Can you work these out from the model? Positions are in its coordinate system, mm. Round coordinates to 2 decimals unless told otherwise and drop trailing zeros. Write each loop counter-clockwise with the first axis right and the second up, starting at its lowest first coordinate (ties: lowest second). Pieces come first, ordered by that corner, then holes. Notation, with made-up numbers: M -15,29.5 L 0,29.5 A25 ccw 0,68.5 Z; hole C 34,-32.75 d10. An arc over 180 degrees is marked long. Answer in a Markdown table with one row per item. Add a question column.
(1) Suppose I cut it at B-B, the plane z = -16.5. Write out the boundary of the cut face in (x, y).
(2) Suppose I cut it at A-A, the plane x = -39. Write out the boundary of the cut face in (y, z), then the cut area to 3 significant figures.
(3) I'm going to push flat-ended pins straight in: pin 1 (1.5 mm diameter, centred on x = 27.5, y = 1, fed in from +Z); pin 2 (1.3 mm diameter, centred on x = -55.5, y = 1, fed in from -Z); pin 3 (1.3 mm diameter, centred on y = 2, z = -1, fed in from -X). Where does each tip first touch, or does it pass through?
(4) If I drill on probe 1 along X at (y, z) = (1.2, -22); probe 2 along X at (y, z) = (1.45, 20.5); probe 3 along Z at (x, y) = (-6, 0.25), over which ranges is the centre line in solid material (lowest first)?
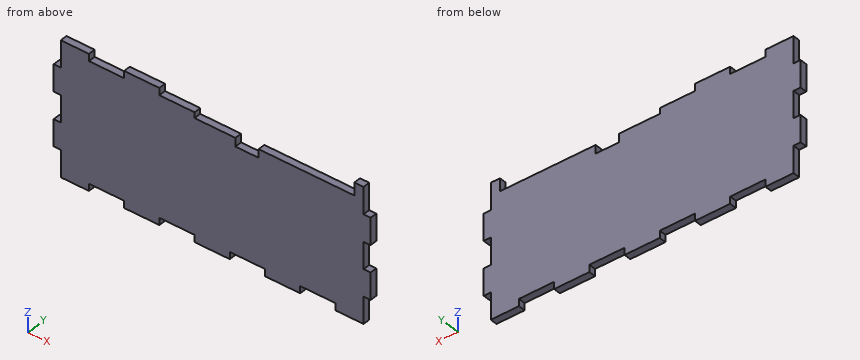
from build123d import *

# Parameters (mm, degrees)
SKETCH1_W           = 114.3
SKETCH1_H           = 48.006
BOSS_EXTRUDE1_DEPTH = 2.54
CUT_EXTRUDE2_REACH  = 64.038
SKETCH2_W           = 2.54
SKETCH2_H           = 9.6012
SKETCH2_W_2         = 12.7
SKETCH2_H_2         = 2.54
CUT_EXTRUDE3_DEPTH  = 2.54


with BuildPart() as part:
    # Sketch1 → Boss-Extrude1 (new body)
    with BuildSketch(Plane(origin=(0, 0, 0), x_dir=(1, 0, 0), z_dir=(0, 1, 0))):
        Rectangle(SKETCH1_W, SKETCH1_H)
    extrude(amount=BOSS_EXTRUDE1_DEPTH)

    # Sketch2 → Cut-Extrude2 (cut, up to next)
    with BuildSketch(Plane(origin=(0, 2.54, 0), x_dir=(1, 0, 0), z_dir=(0, 1, 0)), mode=Mode.PRIVATE) as cut_extrude2_sk1:
        with Locations((-55.88, 19.2024)):
            Rectangle(SKETCH2_W, SKETCH2_H)
    cut_extrude2_tool1 = extrude(cut_extrude2_sk1.sketch, amount=-CUT_EXTRUDE2_REACH, mode=Mode.PRIVATE) & part.part
    # Sketch2 → Cut-Extrude2 (cut, up to next)
    with BuildSketch(Plane(origin=(0, 2.54, 0), x_dir=(1, 0, 0), z_dir=(0, 1, 0)), mode=Mode.PRIVATE) as cut_extrude2_sk2:
        with Locations((-38.1, 22.733)):
            Rectangle(SKETCH2_W_2, SKETCH2_H_2)
    cut_extrude2_tool2 = extrude(cut_extrude2_sk2.sketch, amount=-CUT_EXTRUDE2_REACH, mode=Mode.PRIVATE) & part.part
    # Sketch2 → Cut-Extrude2 (cut, up to next)
    with BuildSketch(Plane(origin=(0, 2.54, 0), x_dir=(1, 0, 0), z_dir=(0, 1, 0)), mode=Mode.PRIVATE) as cut_extrude2_sk3:
        with Locations((-12.7, 22.733)):
            Rectangle(SKETCH2_W_2, SKETCH2_H_2)
    cut_extrude2_tool3 = extrude(cut_extrude2_sk3.sketch, amount=-CUT_EXTRUDE2_REACH, mode=Mode.PRIVATE) & part.part
    # Sketch2 → Cut-Extrude2 (cut, up to next)
    with BuildSketch(Plane(origin=(0, 2.54, 0), x_dir=(1, 0, 0), z_dir=(0, 1, 0)), mode=Mode.PRIVATE) as cut_extrude2_sk4:
        with Locations((12.7, 22.733)):
            Rectangle(SKETCH2_W_2, SKETCH2_H_2)
    cut_extrude2_tool4 = extrude(cut_extrude2_sk4.sketch, amount=-CUT_EXTRUDE2_REACH, mode=Mode.PRIVATE) & part.part
    # Sketch2 → Cut-Extrude2 (cut, up to next)
    with BuildSketch(Plane(origin=(0, 2.54, 0), x_dir=(1, 0, 0), z_dir=(0, 1, 0)), mode=Mode.PRIVATE) as cut_extrude2_sk5:
        with Locations((38.1, 22.733)):
            Rectangle(SKETCH2_W_2, SKETCH2_H_2)
    cut_extrude2_tool5 = extrude(cut_extrude2_sk5.sketch, amount=-CUT_EXTRUDE2_REACH, mode=Mode.PRIVATE) & part.part
    # Sketch2 → Cut-Extrude2 (cut, up to next)
    with BuildSketch(Plane(origin=(0, 2.54, 0), x_dir=(1, 0, 0), z_dir=(0, 1, 0)), mode=Mode.PRIVATE) as cut_extrude2_sk6:
        with Locations((55.88, 19.2024)):
            Rectangle(SKETCH2_W, SKETCH2_H)
    cut_extrude2_tool6 = extrude(cut_extrude2_sk6.sketch, amount=-CUT_EXTRUDE2_REACH, mode=Mode.PRIVATE) & part.part
    # Sketch2 → Cut-Extrude2 (cut, up to next)
    with BuildSketch(Plane(origin=(0, 2.54, 0), x_dir=(1, 0, 0), z_dir=(0, 1, 0)), mode=Mode.PRIVATE) as cut_extrude2_sk7:
        with Locations((55.88, 0)):
            Rectangle(SKETCH2_W, SKETCH2_H)
    cut_extrude2_tool7 = extrude(cut_extrude2_sk7.sketch, amount=-CUT_EXTRUDE2_REACH, mode=Mode.PRIVATE) & part.part
    # Sketch2 → Cut-Extrude2 (cut, up to next)
    with BuildSketch(Plane(origin=(0, 2.54, 0), x_dir=(1, 0, 0), z_dir=(0, 1, 0)), mode=Mode.PRIVATE) as cut_extrude2_sk8:
        with Locations((55.88, -19.2024)):
            Rectangle(SKETCH2_W, SKETCH2_H)
    cut_extrude2_tool8 = extrude(cut_extrude2_sk8.sketch, amount=-CUT_EXTRUDE2_REACH, mode=Mode.PRIVATE) & part.part
    # Sketch2 → Cut-Extrude2 (cut, up to next)
    with BuildSketch(Plane(origin=(0, 2.54, 0), x_dir=(1, 0, 0), z_dir=(0, 1, 0)), mode=Mode.PRIVATE) as cut_extrude2_sk9:
        with Locations((38.1, -22.733)):
            Rectangle(SKETCH2_W_2, SKETCH2_H_2)
    cut_extrude2_tool9 = extrude(cut_extrude2_sk9.sketch, amount=-CUT_EXTRUDE2_REACH, mode=Mode.PRIVATE) & part.part
    # Sketch2 → Cut-Extrude2 (cut, up to next)
    with BuildSketch(Plane(origin=(0, 2.54, 0), x_dir=(1, 0, 0), z_dir=(0, 1, 0)), mode=Mode.PRIVATE) as cut_extrude2_sk10:
        with Locations((12.7, -22.733)):
            Rectangle(SKETCH2_W_2, SKETCH2_H_2)
    cut_extrude2_tool10 = extrude(cut_extrude2_sk10.sketch, amount=-CUT_EXTRUDE2_REACH, mode=Mode.PRIVATE) & part.part
    # Sketch2 → Cut-Extrude2 (cut, up to next)
    with BuildSketch(Plane(origin=(0, 2.54, 0), x_dir=(1, 0, 0), z_dir=(0, 1, 0)), mode=Mode.PRIVATE) as cut_extrude2_sk11:
        with Locations((-12.7, -22.733)):
            Rectangle(SKETCH2_W_2, SKETCH2_H_2)
    cut_extrude2_tool11 = extrude(cut_extrude2_sk11.sketch, amount=-CUT_EXTRUDE2_REACH, mode=Mode.PRIVATE) & part.part
    # Sketch2 → Cut-Extrude2 (cut, up to next)
    with BuildSketch(Plane(origin=(0, 2.54, 0), x_dir=(1, 0, 0), z_dir=(0, 1, 0)), mode=Mode.PRIVATE) as cut_extrude2_sk12:
        with Locations((-38.1, -22.733)):
            Rectangle(SKETCH2_W_2, SKETCH2_H_2)
    cut_extrude2_tool12 = extrude(cut_extrude2_sk12.sketch, amount=-CUT_EXTRUDE2_REACH, mode=Mode.PRIVATE) & part.part
    # Sketch2 → Cut-Extrude2 (cut, up to next)
    with BuildSketch(Plane(origin=(0, 2.54, 0), x_dir=(1, 0, 0), z_dir=(0, 1, 0)), mode=Mode.PRIVATE) as cut_extrude2_sk13:
        with Locations((-55.88, -19.2024)):
            Rectangle(SKETCH2_W, SKETCH2_H)
    cut_extrude2_tool13 = extrude(cut_extrude2_sk13.sketch, amount=-CUT_EXTRUDE2_REACH, mode=Mode.PRIVATE) & part.part
    # Sketch2 → Cut-Extrude2 (cut, up to next)
    with BuildSketch(Plane(origin=(0, 2.54, 0), x_dir=(1, 0, 0), z_dir=(0, 1, 0)), mode=Mode.PRIVATE) as cut_extrude2_sk14:
        with Locations((-55.88, 0)):
            Rectangle(SKETCH2_W, SKETCH2_H)
    cut_extrude2_tool14 = extrude(cut_extrude2_sk14.sketch, amount=-CUT_EXTRUDE2_REACH, mode=Mode.PRIVATE) & part.part
    add(cut_extrude2_tool1.solids().sort_by_distance((-55.88, 2.54, -19.2024))[0], mode=Mode.SUBTRACT)
    add(cut_extrude2_tool2.solids().sort_by_distance((-38.1, 2.54, -22.733))[0], mode=Mode.SUBTRACT)
    add(cut_extrude2_tool3.solids().sort_by_distance((-12.7, 2.54, -22.733))[0], mode=Mode.SUBTRACT)
    add(cut_extrude2_tool4.solids().sort_by_distance((12.7, 2.54, -22.733))[0], mode=Mode.SUBTRACT)
    add(cut_extrude2_tool5.solids().sort_by_distance((38.1, 2.54, -22.733))[0], mode=Mode.SUBTRACT)
    add(cut_extrude2_tool6.solids().sort_by_distance((55.88, 2.54, -19.2024))[0], mode=Mode.SUBTRACT)
    add(cut_extrude2_tool7.solids().sort_by_distance((55.88, 2.54, 0))[0], mode=Mode.SUBTRACT)
    add(cut_extrude2_tool8.solids().sort_by_distance((55.88, 2.54, 19.2024))[0], mode=Mode.SUBTRACT)
    add(cut_extrude2_tool9.solids().sort_by_distance((38.1, 2.54, 22.733))[0], mode=Mode.SUBTRACT)
    add(cut_extrude2_tool10.solids().sort_by_distance((12.7, 2.54, 22.733))[0], mode=Mode.SUBTRACT)
    add(cut_extrude2_tool11.solids().sort_by_distance((-12.7, 2.54, 22.733))[0], mode=Mode.SUBTRACT)
    add(cut_extrude2_tool12.solids().sort_by_distance((-38.1, 2.54, 22.733))[0], mode=Mode.SUBTRACT)
    add(cut_extrude2_tool13.solids().sort_by_distance((-55.88, 2.54, 19.2024))[0], mode=Mode.SUBTRACT)
    add(cut_extrude2_tool14.solids().sort_by_distance((-55.88, 2.54, 0))[0], mode=Mode.SUBTRACT)

    # Sketch5 → Cut-Extrude3 (cut)
    with BuildSketch(Plane(origin=(0, 2.54, 0), x_dir=(1, 0, 0), z_dir=(0, 1, 0))):
        Polygon((16.764, -19.431), (51.308, -19.431), (51.308, -24.003), (-6.35, -24.003), (-6.35, -19.431), (8.382, -19.431), (8.382, -16.383), (16.764, -16.383), align=None)
    extrude(amount=-CUT_EXTRUDE3_DEPTH, mode=Mode.SUBTRACT)


solid = part.part
Calculated:
| question | item | result |
|---|---|---|
| 1 | outline | M -54.61,0 L 54.61,0 L 54.61,2.54 L -54.61,2.54 Z |
| 2 | outline | M 0,-21.46 L 2.54,-21.46 L 2.54,21.46 L 0,21.46 Z |
| 2 | area | 109 mm² |
| 3 | pin 1 | z = 19.43 |
| 3 | pin 2 | z = -14.4 |
| 3 | pin 3 | x = -54.61 |
| 4 | probe 1 | -54.61 to -44.45, -31.75 to -19.05, -6.35 to 6.35, 19.05 to 31.75, 44.45 to 54.61 |
| 4 | probe 2 | -54.61 to -6.35, 51.31 to 54.61 |
| 4 | probe 3 | -24 to 19.43 |
